Geometry: see drawing. Coordinates: mm, zero at the bounding-box minimum. Round coordinates to 2 decimals unless told otherwise and drop trailing zeros.
(1) Section A-A, the plane x = 6.5. Count the separate pieces of the cut face and the enclosed holes in it, plus the area to 3 significant figures.
(2) Mould query, pull axis Y, two halves, no side actions, for the marked faces 1, 2 and 3. Classes: pulls with the +Y half, pulls with the -Y half, needs draft (parallel to the pull), parting line crosses it, or undercut.
(3) First-contact query: pin 1 Ø3 at (x, z) = (5, 3.5) entering from +Y. Flat tip, straight axial feed; report the tip coordinate or a pass-through.
(4) Material intervals for probe 1 along Y at (x, z) = (4, 7.75) (1 decimal); probe 2 along X at (y, z) = (9.5, 4.25) (1 decimal); probe 3 along X at (y, z) = (7.25, 6.75) (1 decimal), sorted ascending.
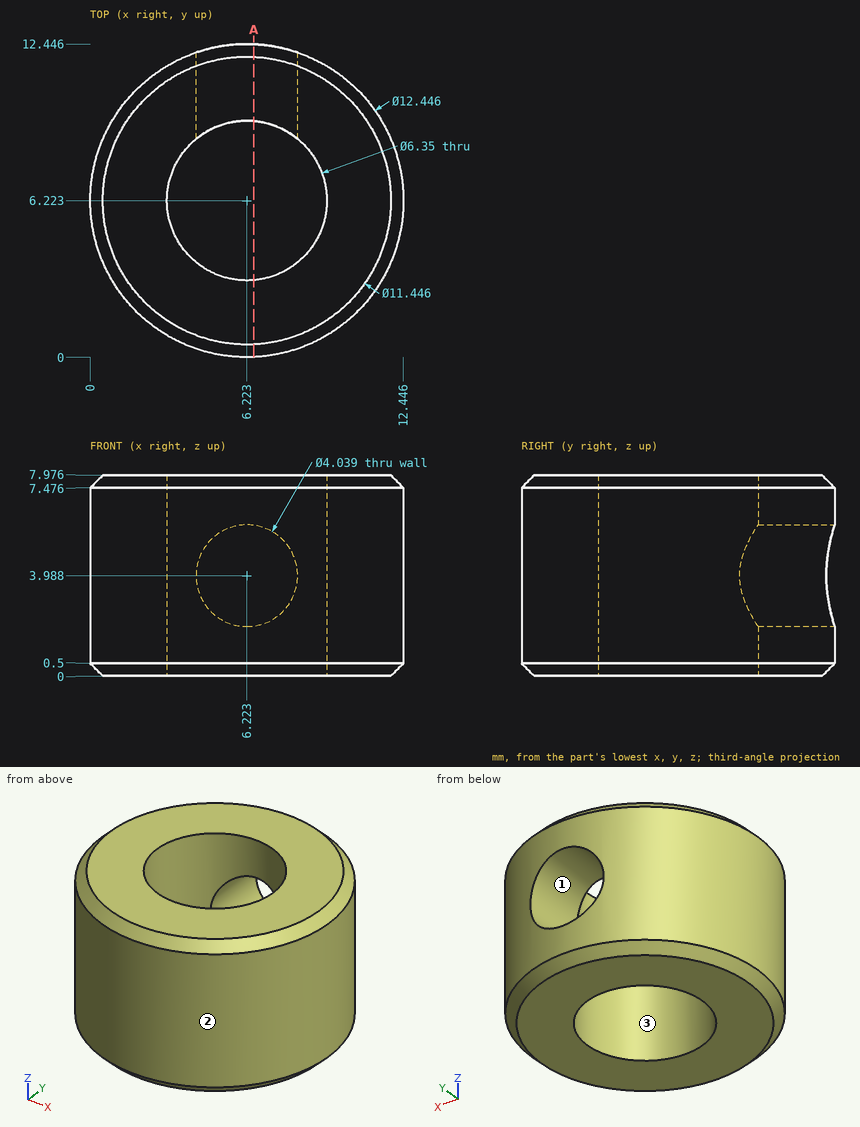
Output values:
1. separate pieces: 3
1. enclosed holes: 0
1. area: 36.0 mm2
2. face 1: needs draft
2. face 2: parting line crosses it
2. face 3: undercut
3. pin 1: stops at y = 12.41
4. probe 1: y = 0.7 to 4, 8.5 to 11.7
4. probe 2: x = 0.9 to 4.2, 8.2 to 11.5
4. probe 3: x = 0.1 to 3.2, 9.2 to 12.4
